```python
from build123d import *

# Parameters (mm, degrees)
BOSS_EXTRUDE1_DEPTH     = 35
CUT_EXTRUDE1_DEPTH      = 45.485952839
CUT_EXTRUDE1_DEPTH_BACK = 45.485952839
SKETCH2_R               = 12.8
SKETCH3_R               = 1.8
CUT_EXTRUDE2_DEPTH      = 16
SKETCH4_R               = 3.25
CUT_EXTRUDE3_DEPTH      = 5.6
CUT_EXTRUDE4_DEPTH      = 45.485953003
CUT_EXTRUDE4_DEPTH_BACK = 45.485953003
SKETCH5_R               = 1.8
SKETCH6_R               = 3.75
CUT_EXTRUDE5_DEPTH      = 5
CUT_EXTRUDE6_DEPTH      = 8


with BuildPart() as part:
    # Sketch1 → Boss-Extrude1 (new, symmetric)
    with BuildSketch(Plane(origin=(0, 0, 0), x_dir=(0, 0, -1), z_dir=(1, 0, 0))):
        with BuildLine():
            Line((-19, -15), (19, -15))
            ThreePointArc((19, -15), (21.828427125, -13.828427125), (23, -11))
            Line((23, -11), (23, -4.6))
            ThreePointArc((23, -4.6), (21.828427125, -1.771572875), (19, -0.6))
            Line((19, -0.6), (-19, -0.6))
            ThreePointArc((-19, -0.6), (-21.828427125, -1.771572875), (-23, -4.6))
            Line((-23, -4.6), (-23, -11))
            ThreePointArc((-23, -11), (-21.828427125, -13.828427125), (-19, -15))
        make_face()
    extrude(amount=BOSS_EXTRUDE1_DEPTH, both=True)

    # Sketch2 → Cut-Extrude1 (cut, two sides: drawn at the far end of the back side and taken through both)
    with BuildSketch(Plane(origin=(0, 0, 0), x_dir=(0, 0, -1), z_dir=(1, 0, 0)).offset(-CUT_EXTRUDE1_DEPTH_BACK)):
        Circle(SKETCH2_R)
    extrude(amount=CUT_EXTRUDE1_DEPTH + CUT_EXTRUDE1_DEPTH_BACK, mode=Mode.SUBTRACT)

    # Sketch3 → Cut-Extrude2 (cut)
    with BuildSketch(Plane(origin=(0, -15, 0), x_dir=(1, 0, 0), z_dir=(0, 1, 0))):
        with Locations(Location((28, -17.5, 0), (0, 0, 236.442690238))):
            Circle(SKETCH3_R)
        with Locations(Location((28, 17.5, 0), (0, 0, 123.557309762))):
            Circle(SKETCH3_R)
        with Locations(Location((-28, -17.5, 0), (0, 0, 236.442690238))):
            Circle(SKETCH3_R)
        with Locations(Location((-28, 17.5, 0), (0, 0, 123.557309762))):
            Circle(SKETCH3_R)
    extrude(amount=CUT_EXTRUDE2_DEPTH, mode=Mode.SUBTRACT)

    # Sketch4 → Cut-Extrude3 (cut)
    with BuildSketch(Plane(origin=(0, -15, 0), x_dir=(1, 0, 0), z_dir=(0, 1, 0))):
        with Locations(Location((28, -17.5, 0), (0, 0, 207.48642625))):
            Circle(SKETCH4_R)
        with Locations(Location((28, 17.5, 0), (0, 0, 27.48642625))):
            Circle(SKETCH4_R)
        with Locations(Location((-28, -17.5, 0), (0, 0, 207.48642625))):
            Circle(SKETCH4_R)
        with Locations(Location((-28, 17.5, 0), (0, 0, 27.48642625))):
            Circle(SKETCH4_R)
    extrude(amount=CUT_EXTRUDE3_DEPTH, mode=Mode.SUBTRACT)

    # Sketch5 → Cut-Extrude4 (cut, two sides: drawn at the far end of the back side and taken through both)
    with BuildSketch(Plane.XY.offset(-CUT_EXTRUDE4_DEPTH_BACK)):
        with Locations((18, 0)):
            Circle(SKETCH5_R)
        with Locations((-18, 0)):
            Circle(SKETCH5_R)
    extrude(amount=CUT_EXTRUDE4_DEPTH + CUT_EXTRUDE4_DEPTH_BACK, mode=Mode.SUBTRACT)

    # Sketch6 → Cut-Extrude5 (cut)
    with BuildSketch(Plane.XY.offset(23)):
        with Locations((18, 0)):
            Circle(SKETCH6_R)
        with Locations((-18, 0)):
            Circle(SKETCH6_R)
    extrude(amount=-CUT_EXTRUDE5_DEPTH, mode=Mode.SUBTRACT)

    # Sketch7 → Cut-Extrude6 (cut)
    with BuildSketch(Plane.XY.offset(-23)):
        Polygon((20.85, 1.645448267), (18, 3.290896534), (15.15, 1.645448267), (15.15, -1.645448267), (18, -3.290896534), (20.85, -1.645448267), align=None)
        Polygon((-15.15, 1.645448267), (-18, 3.290896534), (-20.85, 1.645448267), (-20.85, -1.645448267), (-18, -3.290896534), (-15.15, -1.645448267), align=None)
    extrude(amount=CUT_EXTRUDE6_DEPTH, mode=Mode.SUBTRACT)


solid = part.part
```
Design review of the part built by this model. Coordinates are the model's own, in mm. A direction names the side the tool comes from. Coordinates: 2 decimals unless noted, no trailing zeros. Order: outer loops, then holes, each group sorted by start corner. A loop starts at its lowest first (then second) coordinate and runs counter-clockwise, first axis right, second up. Notation, with made-up numbers: (-16, 44.25) - (20, 44.25) arc R18 ccw to (20, 51.25) - close; hole circle Ø6 at (-3.5, -13.5). An arc over 180 degrees is marked (long way). One line per question, with ' | ' between items.
Q1. Consider section D-D, the plane x = 28. Give the boundary of the cut face in (y, z), then the cut area to 3 significant figures.
Answer key:
outline: (-15, -14.25) - (-9.4, -14.25) - (-9.4, -15.7) - (-0.6, -15.7) - (-0.6, -12.79) arc R12.8 cw to (-0.6, 12.79) - (-0.6, 15.7) - (-9.4, 15.7) - (-9.4, 14.25) - (-15, 14.25) - close; (-14.6, -20.75) arc R4 ccw to (-11, -23) - (-4.6, -23) arc R4 ccw to (-0.61, -19.3) - (-9.4, -19.3) - (-9.4, -20.75) - close; (-14.6, 20.75) - (-9.4, 20.75) - (-9.4, 19.3) - (-0.61, 19.3) arc R4 ccw to (-4.6, 23) - (-11, 23) arc R4 ccw to start | area: 271 mm2
Q2. For faces 1 (the cylindrical face through (28.84, -12.24, -14.36)), 2 (the flat face through (0, -0.6, -16)), 3 (the cylindrical face through (0.49, -13.797, 21.859)), 4 (the flat face through (-19.44, -2.46, -18.94)), 5 (the cylindrical face through (17.93, -3.75, 20.49)), list the 3-axis set-ups (+Z, -Z, +X, -X, +Y, -Y) from which the entire face can be reached by the end or side of a thin tool; tool diameter is ignored.
Answer key:
face 1: -Y | face 2: +Z, -Z, +X, -X, +Y | face 3: +Z, +X, -X, -Y | face 4: -Z, +Y | face 5: +Z, +Y
Q3. Consider section B-B, the plane x = -11.5. Give the boundary of the cut face in (y, z).
Answer key:
outline: (-15, -19) arc R4 ccw to (-11, -23) - (-4.6, -23) arc R4 ccw to (-0.6, -19) - (-0.6, -12.79) arc R12.8 cw to (-0.6, 12.79) - (-0.6, 19) arc R4 ccw to (-4.6, 23) - (-11, 23) arc R4 ccw to (-15, 19) - close
Q4. Consider section C-C, the plane y = -14. Give the boundary of the cut face in (x, z).
Answer key:
outline: (-35, -21.65) - (35, -21.65) - (35, 21.65) - (-35, 21.65) - close; hole circle Ø6.5 at (-28, -17.5); hole circle Ø6.5 at (-28, 17.5); hole circle Ø6.5 at (28, -17.5); hole circle Ø6.5 at (28, 17.5)
Q5. To check wall thickness, follow line 1 along X through (y, z) = (-4.5, -17.5); line 2 along X through (y, z) = (-13.55, -17.5); line 3 along Z through (x, y) = (28, -11.3). State the ranges of each line that lie inside material, in increasing order.
Answer key:
line 1: x = -35 to -29.8, -26.2 to 26.2, 29.8 to 35 | line 2: x = -35 to -31.25, -24.75 to 24.75, 31.25 to 35 | line 3: z = -22.99 to -20.75, -14.25 to -6.01, 6.01 to 14.25, 20.75 to 22.99
Q6. Consider section A-A, the plane z = -17.5. Give the number of separate pieces and of enclosed holes in the cut face, then the cut area to 3 significant figures.
Answer key:
separate pieces: 3 | enclosed holes: 0 | area: 851 mm2
Q7. Clearance check with flat-ended pins moving along their axes: pin 1 Ø3 at (x, y) = (17.5, -2) entering from -Z; pin 2 Ø6 at (x, z) = (21.5, 3.5) entering from +Y; pin 3 Ø2 at (x, z) = (-28, 17.5) entering from -Y; pin 4 Ø4 at (x, z) = (-28, -17.5) entering from -Y. State where each tip first meets the part, or that it passes through.
Answer key:
pin 1: stops at z = -22.85 | pin 2: stops at y = -11.03 | pin 3: passes through | pin 4: stops at y = -9.4
